Check sheet for the modelled part. Datum: model origin and axes. Units: mm. A direction names the side the tool comes from. Coordinates: 2 decimals unless noted, no trailing zeros. Loops run counter-clockwise (first coordinate to the right, second up) from the corner with the lowest first, then second, coordinate; pieces in that order, holes last. Notation, with made-up numbers: (-36, 40) - (-22, 40) arc R24 cw to (-22, 53) - close; hole circle Ø7 at (66, 54.5). An arc over 180 degrees is marked (long way). Write each question's results on one line, items separated by ' | '. Start each with the question number.
1. Cross-section at C-C (z = 5). Record the cut outline in (x, y) (3 decimals).
2. Gauge pin test, flat ends, axial feed: P1, Ø7.5, axis at x = -54.5, z = 10, coming from the -Y side; P2, Ø1.5, axis at y = 2, z = 7.5, coming from the +X side; P3, Ø3.5, axis at x = -35.5, z = 25.5, coming from the -Y side. Record the tip position at first contact, or that the pin passes through.
3. Tool access check on faces 5 (the face through (-46.35, 3.45, 38.77)), 6 (the face through (-69.973, 1.653, 28.64)), 7 (the face through (-38.375, 2, 8)), 8 (the face through (-51, 3, 38.5)), 9 (the face through (-51, 7, 21)). Record the directions out of +Z, -Z, +X, -X, +Y, -Y that give a thin tool (end or side, any length) a straight path to the whole face; none if there is none.
4. Cross-section at B-B (y = 0.75). Give the number of separate pieces and of enclosed holes in the cut face, and give its area (3 significant figures).
5. Cross-section at D-D (z = 9.5). Record the cut outline in (x, y) (3 decimals), and give its area (3 significant figures).
6. Draft check along Z on faces 1 (the face through (-26, 0, 22)), 2 (the face through (-30.4, 3.45, 40.61)), 3 (the face through (-53.475, 3.451, 37.022)), 4 (the face through (-50.6, 2.46, 26.37)). Enter one of: released by +Z, released by -Z, zero draft, split by the parting line, or undercut.
7. Thickness scan on line 1 (X direction, y = 1.75, z = 4) (3 decimals); line 2 (X direction, y = 2, z = 8) (3 decimals); line 3 (Y direction, x = -61, z = 19.5). Record the ranges inside material, lowest first. Write a range as [from, to].
Autodesk Inventor part; units mm, degrees
ref_plane "YZ Plane" through (0, 0, 0) normal (1, 0, 0) x (0, 1, 0)
ref_plane "XZ Plane" through (0, 0, 0) normal (0, 1, 0) x (-1, 0, 0)
ref_plane "XY Plane" through (0, 0, 0) normal (0, 0, 1) x (1, 0, 0)
sketch "スケッチ1" plane through (0, 0, 0) normal (0, 1, 0) x (-1, 0, 0)
  arc A0 (54.8142, 37.6946) -> (46.9358, 37.6946) centre (50.875, 37) ccw
  circle A1 centre (50.875, 13.875) radius 12.5
  line L0 (50.875, 37) -> (87.3129, 43.425)
  line L1 (50.875, 37) -> (87.875, 37) construction
  line L2 (87.3129, 43.425) -> (50.875, 37)
  line L3 (50.875, 37) -> (14.4371, 43.425)
  arc A2 (13.4523, 43.5986) -> (88.2977, 43.5986) centre (50.875, 37) ccw
  line L4 (87.3129, 43.425) -> (88.2977, 43.5986)
  line L5 (13.4523, 43.5986) -> (14.4371, 43.425)
  point P0 (0, 0)
  dimension "d22" = 25
  dimension "d27" = 10
  dimension "d38" = 4
  dimension "d49" = 76
extrude "押し出し1" add sketch "スケッチ1" along normal blind 7
sketch "スケッチ2" plane through (0, 7, 0) normal (0, 1, 0) x (1, 0, 0)
  circle A0 centre (-50.875, -13.875) radius 12.5
  circle A1 centre (-50.875, -13.875) radius 12.5
  point P0 (0, 0)
extrude "押し出し2" add sketch "スケッチ2" against normal blind 2
sketch "スケッチ3" plane through (0, 0, 0) normal (0, -1, 0) x (1, 0, 0)
  circle A0 centre (-50.875, 13.875) radius 12.5
  circle A1 centre (-50.875, 13.875) radius 12.5
  line L0 (-63.375, 13.875) -> (-38.375, 13.875)
  line L1 (-38.375, 13.875) -> (-38.375, -3.3785)
  line L2 (-38.375, -3.3785) -> (-63.375, -3.3785)
  line L3 (-63.375, -3.3785) -> (-63.375, 13.875)
  line L4 (-46.9358, 37.6946) -> (-13.4523, 43.5986)
  line L5 (-88.2977, 43.5986) -> (-54.8142, 37.6946)
  arc A2 (-88.2977, 43.5986) -> (-13.4523, 43.5986) centre (-50.875, 37) ccw
  arc A3 (-46.9358, 37.6946) -> (-54.8142, 37.6946) centre (-50.875, 37) ccw
  point P0 (0, 0)
extrude "押し出し3" cut sketch "スケッチ3" against normal blind 5 contours L1 A2 L3 A0 | A0 L0 | L1 L2 L3 A2 picked at (-53.2419, 10.4459)
sketch "スケッチ4" plane through (0, 0, 0) normal (0, -1, 0) x (1, 0, 0)
  circle A0 centre (-50.875, 37) radius 2.6
  arc A1 (-38.375, 13.875) -> (-63.375, 13.875) centre (-50.875, 13.875) ccw
  line L0 (-63.375, 1.1148) -> (-63.375, 13.875)
  line L1 (-38.375, 13.875) -> (-38.375, 1.1148)
  line L2 (-46.9358, 37.6946) -> (-13.4523, 43.5986)
  line L3 (-52.9987, 38.5) -> (-48.7513, 38.5)
  line L4 (-42.875, 38.5) -> (-42.875, 38.4106)
  line L5 (-48.7513, 35.5) -> (-52.9987, 35.5)
  line L6 (-58.875, 38.4106) -> (-58.875, 38.5)
  arc A2 (-38.375, 1.1148) -> (-13.4523, 43.5986) centre (-50.875, 37) ccw
  line L7 (-88.2977, 43.5986) -> (-54.8142, 37.6946)
  arc A3 (-88.2977, 43.5986) -> (-63.375, 1.1148) centre (-50.875, 37) ccw
  arc A4 (-46.9358, 37.6946) -> (-54.8142, 37.6946) centre (-50.875, 37) ccw
  point P0 (0, 0)
  dimension "d12" = 5.2
  dimension "d47" = 3
extrude "押し出し4" cut sketch "スケッチ4" against normal blind 8 contours A0 L5 L3
chamfer "面取り1" distance 2 angle 45 4 edges at (-88.2977, 3.5, 43.5986) (-46.9358, 3.5, 37.6946) (-13.4523, 3.5, 43.5986) (-54.8142, 3.5, 37.6946)
sketch "スケッチ8" plane through (0, 7, 0) normal (0, 1, 0) x (1, 0, 0)
  line L0 (-44.9662, -38.0419) -> (-15.4219, -43.2513)
  arc A0 (-48.7513, -38.5) -> (-48.7513, -35.5) centre (-50.875, -37) ccw
  arc A1 (-13.157, -41.6206) -> (-88.593, -41.6206) centre (-50.875, -37) ccw
  line L1 (-86.3281, -43.2513) -> (-56.7838, -38.0419)
  arc A2 (-52.9987, -35.5) -> (-52.9987, -38.5) centre (-50.875, -37) ccw
  line L2 (-52.9987, -35.5) -> (-48.7513, -35.5)
  line L3 (-48.7513, -38.5) -> (-52.9987, -38.5)
  arc A3 (-53.9856, -39.5148) -> (-47.7644, -39.5148) centre (-50.875, -37) ccw
  line L4 (-13.157, -41.6206) -> (-15.4219, -43.2513)
  line L5 (-86.3281, -43.2513) -> (-88.593, -41.6206)
  line L6 (-53.9856, -39.5148) -> (-56.7838, -38.0419)
  line L7 (-44.9662, -38.0419) -> (-47.7644, -39.5148)
  point P0 (0, 0)
extrude "押し出し8" cut sketch "スケッチ8" along normal blind 0.5 contours L3 A2 L2 A0
sketch "スケッチ9" plane through (0, 0, 0) normal (0, -1, 0) x (1, 0, 0)
  line L0 (-48.7513, 35.5) -> (-52.9987, 35.5)
  arc A0 (-52.9987, 38.5) -> (-52.9987, 35.5) centre (-50.875, 37) ccw
  arc A1 (-48.7513, 35.5) -> (-48.7513, 38.5) centre (-50.875, 37) ccw
  line L1 (-44.9662, 38.0419) -> (-15.4219, 43.2513)
  line L2 (-63.375, 1.1148) -> (-63.375, 13.875)
  arc A2 (-38.375, 13.875) -> (-63.375, 13.875) centre (-50.875, 13.875) ccw
  line L3 (-38.375, 13.875) -> (-38.375, 1.1148)
  circle A3 centre (-50.875, 37) radius 17.5
  circle A4 centre (-50.875, 37) radius 20.5
  circle A5 centre (-50.875, 37) radius 19
  line L4 (-86.3281, 43.2513) -> (-56.7838, 38.0419)
  arc A6 (-88.593, 41.6206) -> (-63.375, 1.1148) centre (-50.875, 37) ccw
  arc A7 (-38.375, 1.1148) -> (-13.157, 41.6206) centre (-50.875, 37) ccw
  line L5 (-52.9987, 38.5) -> (-48.7513, 38.5)
  arc A8 (-47.7644, 39.5148) -> (-53.9856, 39.5148) centre (-50.875, 37) ccw
  line L6 (-15.4219, 43.2513) -> (-13.157, 41.6206)
  line L7 (-47.7644, 39.5148) -> (-44.9662, 38.0419)
  line L8 (-56.7838, 38.0419) -> (-53.9856, 39.5148)
  line L9 (-88.593, 41.6206) -> (-86.3281, 43.2513)
  point P0 (0, 0)
  dimension "d39" = 35
  dimension "d40" = 41
  dimension "d41" = 38
extrude "押し出し9" cut sketch "スケッチ9" against normal blind 2 contours L0 A0 L5 A1 | A3 L4 A5 L1 | L1 A5 A2 A3 | A5 L4 A4 L1 | L1 A4 A2 A5 | A3 A2 A5 L4 | A5 A2 A4 L4 | A2 A5 A3 | A2 A4 A5
chamfer "面取り2" distance 2 angle 45 4 edges at (-69.646, 0, 28.7598) (-32.104, 0, 28.7598) (-66.8754, 0, 29.9123) (-34.8746, 0, 29.9123)
properties part number "RescueKitThrow-Joint"
Established:
1) outline: (-71.369, 0) - (-63.375, 0) - (-63.375, 5) - (-38.375, 5) - (-38.375, 0) - (-30.381, 0) - (-30.381, 7) - (-71.369, 7) - close
2) P1: y = 5 | P2: x = -26.03 | P3: y = 1.55
3) face 5: +Z, +Y, -Y | face 6: -Y | face 7: -Z, -Y | face 8: +Y, -Y | face 9: +Z, -Z, +X, -X, +Y
4) separate pieces: 3 | enclosed holes: 1 | area: 1,680 mm^2
5) outline: (-77.1, 0) - (-63.375, 0) - (-63.375, 5) - (-38.375, 5) - (-38.375, 0) - (-24.65, 0) - (-24.65, 7) - (-77.1, 7) - close | area: 242 mm^2
6) face 1: zero draft | face 2: released by +Z | face 3: undercut | face 4: released by -Z
7) line 1: [-69.716, -63.375], [-38.375, -32.034] | line 2: [-75.431, -63.375], [-38.375, -26.319] | line 3: [5, 7]
